Autodesk Inventor part; units mm, degrees
ref_plane "YZ Plane" through (0, 0, 0) normal (1, 0, 0) x (0, 1, 0)
ref_plane "XZ Plane" through (0, 0, 0) normal (0, 1, 0) x (-1, 0, 0)
ref_plane "XY Plane" through (0, 0, 0) normal (0, 0, 1) x (1, 0, 0)
sketch "Esboço1" plane through (0, 0, 0) normal (0, 0, 1) x (1, 0, 0)
  line L0 (-50.5, -37) -> (50.5, -37)
  line L1 (50.5, -37) -> (50.5, 37)
  line L2 (50.5, 37) -> (-50.5, 37)
  line L3 (-50.5, 37) -> (-50.5, -37)
  point P0 (0, 0)
  dimension "d2" = 101
  dimension "d3" = 74
  dimension "d4" = 101
  dimension "d5" = 50.5
  dimension "d6" = 37
extrude "Extrusão1" add sketch "Esboço1" against normal blind 2
sketch "Esboço2" plane through (0, 0, 0) normal (0, 0, 1) x (1, 0, 0)
  line L0 (-50.5, -37) -> (-50.5, 37)
  line L1 (-50.5, 37) -> (50.5, 37)
  line L2 (-46.5, 37) -> (-46.5, -37) construction
  line L3 (50.5, -37) -> (-50.5, -37)
  line L4 (46.5, 37) -> (46.5, -37) construction
  line L5 (-50.5, 18.5) -> (50.5, 18.5) construction
  line L6 (-50.5, -18.5) -> (50.5, -18.5) construction
  line L7 (50.5, 37) -> (50.5, -37)
  point P0 (0, 0)
  point P1 (-46.5, 18.5)
  point P2 (-46.5, -18.5)
  point P3 (46.5, -18.5)
  point P4 (46.5, 18.5)
  dimension "d13" = 4
  dimension "d14" = 97
  dimension "d15" = 18.5
  dimension "d16" = 55.5
  dimension "d17" = 0
hole "Furo1" at (-46.5, 18.5, 0) at (-46.5, -18.5, 0) at (46.5, -18.5, 0) at (46.5, 18.5, 0) direction (0, 0, -1) diameter 2.459 end through all counterbore diameter 6.5 counterbore depth 1.5
properties part number "Ra-Manager_Painel-Placas_Tras_Cego"
Geometry: final body of the model. Coordinates: model frame, mm. A direction names the side the tool comes from. Coordinates: 2 decimals unless noted, no trailing zeros. Order: outer loops, then holes, each group sorted by start corner. A loop starts at its lowest first (then second) coordinate and runs counter-clockwise, first axis right, second up.
1) Section C-C (z = -0.3). Return loops of the section in (x, y).
Result sheet:
outline: (-50.5, -37) - (50.5, -37) - (50.5, 37) - (-50.5, 37) - close; hole circle Ø6.5 at (-46.5, -18.5); hole circle Ø6.5 at (-46.5, 18.5); hole circle Ø6.5 at (46.5, -18.5); hole circle Ø6.5 at (46.5, 18.5)
2) Ray query, probe 1 along X at (y, z) = (18.5, -1); probe 2 along Y at (x, z) = (-46.5, -1.8); probe 3 along X at (y, z) = (18.5, -1.7). Return the intervals inside material, ascending.
Result sheet:
probe 1: x = -50.5 to -49.75, -43.25 to 43.25, 49.75 to 50.5
probe 2: y = -37 to -19.73, -17.27 to 17.27, 19.73 to 37
probe 3: x = -50.5 to -47.73, -45.27 to 45.27, 47.73 to 50.5
3) Section B-B (y = -18.5). Return loops of the section in (x, z), then the cut area to 3 significant figures.
Result sheet:
outline: (-50.5, -2) - (-47.73, -2) - (-47.73, -1.5) - (-49.75, -1.5) - (-49.75, 0) - (-50.5, 0) - close; (-45.27, -2) - (45.27, -2) - (45.27, -1.5) - (43.25, -1.5) - (43.25, 0) - (-43.25, 0) - (-43.25, -1.5) - (-45.27, -1.5) - close; (47.73, -2) - (50.5, -2) - (50.5, 0) - (49.75, 0) - (49.75, -1.5) - (47.73, -1.5) - close
area: 180 mm2
4) Set-up query: faces 4 (the cylindrical face through (49.673, -17.795, -0.76)), 5 (the flat face through (-1, 1, -2)). Return all of +Z, -Z, +X, -X, +Y, -Y with unobstructed straight access to the full face (end or side cutting, diameter ignored); none if empty.
Result sheet:
face 4: +Z
face 5: -Z, +X, -X, +Y, -Y
5) Draft query along X for faces 1 (the flat face through (-50.5, 1, -1)), 2 (the flat face through (1, 37, -1)), 3 (the cylindrical face through (45.463, -19.161, -1.754)). Return one class per face: released by +X, released by -X, zero draft, split by the parting line, or undercut.
Result sheet:
face 1: released by -X
face 2: zero draft
face 3: undercut
6) First-contact query: P1, Ø4, axis at x = 46.5, y = 18.5, coming from the +Z side; P2, Ø1.5, axis at x = -46.5, y = -18.5, coming from the -Z side. Flat tips, straight axial feed; report the tip coordinate or a pass-through.
Result sheet:
P1: stops at z = -1.5
P2: passes through
7) Section A-A (x = 46.5). Return loops of the section in (y, z).
Result sheet:
outline: (-37, -2) - (-19.73, -2) - (-19.73, -1.5) - (-21.75, -1.5) - (-21.75, 0) - (-37, 0) - close; (-17.27, -2) - (17.27, -2) - (17.27, -1.5) - (15.25, -1.5) - (15.25, 0) - (-15.25, 0) - (-15.25, -1.5) - (-17.27, -1.5) - close; (19.73, -2) - (37, -2) - (37, 0) - (21.75, 0) - (21.75, -1.5) - (19.73, -1.5) - close
